For this review, take the finished solid that the model builds, in its own axes (mm). A direction names the side the tool comes from. Give positions to 0.01 mm unless a question says otherwise; leave off trailing zeros. Order: outer loops, then holes, each group sorted by start corner. A loop starts at its lowest first (then second) coordinate and runs counter-clockwise, first axis right, second up. Notation, with made-up numbers: M 33.25,17.25 L 71.25,17.25 A30 ccw 71.25,43.25 Z; hole C 13.5,9.5 d4. An arc over 180 degrees is marked long. Use CSV: the item, a comma, the result in double quotes. Start each with the question number.
(1) Wall thickness on L1, parallel to X at y = 0, z = -17.25; L2, parallel to Z at x = 12, y = -5.5: over which ranges is each line inside the solid? List them lowest first. Write a range as from..to.
(2) Consider section B-B (y = 0). Write out the cut boundary in (x, z).
(3) Tool access review of faces 1 (the face through (8, -19, 2.5)), 2 (the face through (0, 0, 0)), 3 (the face through (-18, 6, -25)): name each direction out of +Z, -Z, +X, -X, +Y, -Y from which nothing blocks a thin tool from reaching the whole face with its end or side.
(4) Consider section A-A (z = 14). Write out the cut boundary in (x, y), and give its area (3 significant figures).
(5) Clearance check with flat-ended pins moving along their axes: P1, Ø11, axis at x = 5.5, y = -9, coming from the +Z side; P2, Ø10, axis at y = 4.5, z = -1, coming from the +X side; P3, Ø10, axis at y = 13.5, z = -0.5, coming from the -X side; P4, Ø6, axis at x = 7, z = 2.5, coming from the +Y side. State where each tip first meets the part, or that it passes through.
(6) Draft analysis for pull direction Y (two halves, no side actions). For faces 4 (the face through (-18, -6, 27.5)), 5 (the face through (-4.01, 18.06, -12.32)), 6 (the face through (-14.6, 13.3, 14.8)), state which applies: pulls with the +Y half, pulls with the -Y half, needs draft (parallel to the pull), parting line crosses it, or undercut.
```python
from build123d import *

# Parameters (mm, degrees)
F0_R     = 21
F1_DEPTH = 2.5
F3_R     = 19.75
F3_R_2   = 18.5
F4_DEPTH = 25
F6_R     = 19.75
F6_R_2   = 18.5
F7_DEPTH = 25


with BuildPart() as f1:
    # F0 (on Top) → F1 (new body)
    with BuildSketch(Plane.XY):
        Circle(F0_R)
    extrude(amount=F1_DEPTH)

    # F3 (on face) → F4 (join)
    with BuildSketch(Plane(origin=(0, 0, 0), x_dir=(1, 0, 0), z_dir=(0, 0, -1))):
        Circle(F3_R)
        Circle(F3_R_2, mode=Mode.SUBTRACT)
    extrude(amount=F4_DEPTH)

    # F6 (on face) → F7 (join)
    with BuildSketch(Plane.XY.offset(2.5)):
        Circle(F6_R)
        Circle(F6_R_2, mode=Mode.SUBTRACT)
    extrude(amount=F7_DEPTH)


solid = f1.part
```
Check result:
1,L1,"x = -19.75..-18.5, 18.5..19.75"
1,L2,"z = 0..2.5"
2,outline,"M -21,0 L -19.75,0 L -19.75,-25 L -18.5,-25 L -18.5,0 L 18.5,0 L 18.5,-25 L 19.75,-25 L 19.75,0 L 21,0 L 21,2.5 L 19.75,2.5 L 19.75,27.5 L 18.5,27.5 L 18.5,2.5 L -18.5,2.5 L -18.5,27.5 L -19.75,27.5 L -19.75,2.5 L -21,2.5 Z"
3,face 1,"+Z"
3,face 2,"-Z"
3,face 3,"-Z, +X, -X, +Y, -Y"
4,outline,"C 0,0 d39.5; hole C 0,0 d37"
4,area,"150 mm^2"
5,P1,"stops at z = 2.5"
5,P2,"stops at x = 21"
5,P3,"stops at x = -19.19"
5,P4,"stops at y = 20.62"
6,face 4,"needs draft"
6,face 5,"undercut"
6,face 6,"parting line crosses it"
